Answer from the drawing. Dimensions are ordinates in mm from the lowest x, y and z of the part. A direction names the side the tool comes from. Coordinates: 2 decimals unless noted, no trailing zeros. Write each loop counter-clockwise with the first axis right and the second up, starting at its lowest first coordinate (ties: lowest second). Pieces come first, ordered by that corner, then holes. Notation, with made-up numbers: (6, 76) -> (24, 76) arc R18 cw to (24, 94) -> close; hole circle Ø10 at (62, -40). An arc over 180 degrees is marked (long way). Return JSON: item names as keys, results as strings.
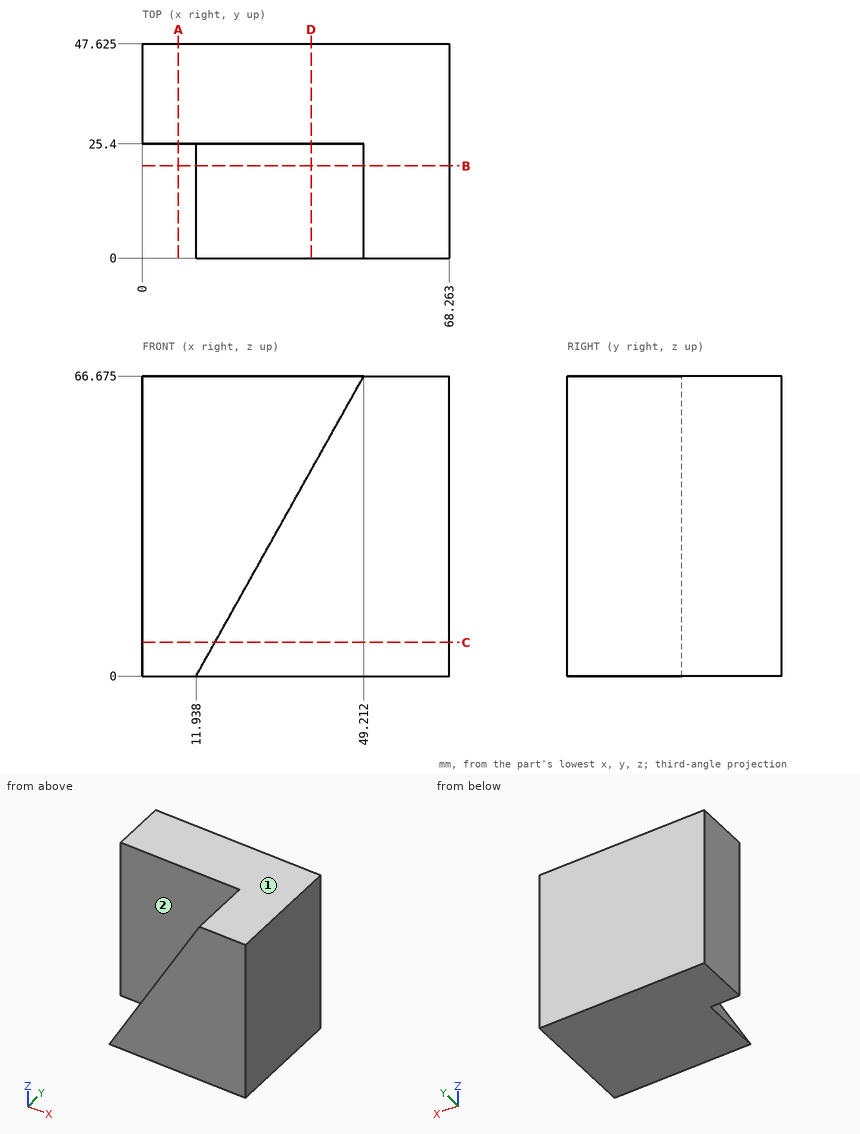
1. A tool of negligible diameter and unlimited length cuts with its end or side. For the marked faces 1 and 2, from which of +Z, -Z, +X, -X, +Y, -Y can it reach the whole face along a straight path? Write none if from no direction.
Taken from the geometry:
{"face 1": "+Z, +X, -X, +Y, -Y", "face 2": "+Z, -X, -Y"}
2. The part is cut by section B-B (y = 20.5). Determine the outline of the cut face in (x, z) (1 decimal), then the cut area to 3 significant figures.
Taken from the geometry:
{"outline": "(11.9, 0) -> (68.3, 0) -> (68.3, 66.7) -> (49.2, 66.7) -> close", "area": "2,510 mm2"}
3. Flat-ended cylindrical pins translate along their axes: pin 1 Ø12 at (x, y) = (47.5, 5) entering from -Z; pin 2 Ø3 at (y, z) = (17, 41.5) entering from -X. Find the tip coordinate at first contact, or state that the pin passes through.
Taken from the geometry:
{"pin 1": "stops at z = 0", "pin 2": "stops at x = 34.3"}
4. Consider L1, parallel to Y at x = 16, z = 23.5 (1 decimal); L2, parallel to Z at x = 31, y = 13.5 (1 decimal); L3, parallel to X at y = 5.5, z = 43 (1 decimal). Determine where each line is inside the solid, lowest interval first.
Taken from the geometry:
{"L1": "y = 25.4 to 47.6", "L2": "z = 0 to 34.1", "L3": "x = 36 to 68.3"}
5. The part is cut by section A-A (x = 8). Determine the outline of the cut face in (y, z) (1 decimal).
Taken from the geometry:
{"outline": "(25.4, 0) -> (47.6, 0) -> (47.6, 66.7) -> (25.4, 66.7) -> close"}
6. The part is cut by section C-C (z = 7.5). Determine the outline of the cut face in (x, y) (1 decimal).
Taken from the geometry:
{"outline": "(0, 25.4) -> (16.1, 25.4) -> (16.1, 0) -> (68.3, 0) -> (68.3, 47.6) -> (0, 47.6) -> close"}
7. The part is cut by section D-D (x = 37.5). Determine the outline of the cut face in (y, z) (1 decimal), then the cut area to 3 significant figures.
Taken from the geometry:
{"outline": "(0, 0) -> (47.6, 0) -> (47.6, 66.7) -> (25.4, 66.7) -> (25.4, 45.7) -> (0, 45.7) -> close", "area": "2,640 mm2"}
